Autodesk Fusion 360 part; units mm, degrees
sketch "base plate" plane through (0, 0, 0) normal (0, 0, 1) x (1, 0, 0)
  line L0 (-228.6, 228.6) -> (228.6, 228.6)
  line L1 (228.6, 228.6) -> (228.6, -228.6)
  line L2 (228.6, -228.6) -> (-228.6, -228.6)
  line L3 (-228.6, -228.6) -> (-228.6, 228.6)
  line L4 (-228.6, 228.6) -> (228.6, -228.6) construction
  line L5 (228.6, 228.6) -> (-228.6, -228.6) construction
  dimension "d1" = 457.2
  dimension "d2" = 457.2
extrude "Extrude1" add sketch "base plate" along normal blind 12.7 makes body 1
sketch "cylinder components" plane through (0, 0, 12.7) normal (0, 0, 1) x (-1, 0, 0)
  line L0 (228.6, 228.6) -> (-228.6, 228.6)
  line L1 (-228.6, 228.6) -> (-228.6, -228.6)
  line L2 (-228.6, -228.6) -> (228.6, -228.6)
  line L3 (228.6, -228.6) -> (228.6, 228.6)
  line L4 (25.4, -114.3) -> (-50.8, -114.3)
  line L5 (-50.8, -114.3) -> (-50.8, 76.2)
  line L6 (-50.8, 76.2) -> (25.4, 76.2)
  line L7 (25.4, 76.2) -> (25.4, -114.3)
  line L8 (-168.91, -76.2) -> (-226.06, -76.2)
  line L9 (-226.06, -76.2) -> (-226.06, -19.05)
  line L10 (-226.06, -19.05) -> (-168.91, -19.05)
  line L11 (-168.91, -19.05) -> (-168.91, -76.2)
  line L12 (0, -254) -> (0, 228.6) construction
  line L13 (25.4, 114.3) -> (-31.75, 114.3)
  line L14 (-31.75, 114.3) -> (-31.75, 171.45)
  line L15 (-31.75, 171.45) -> (25.4, 171.45)
  line L16 (25.4, 171.45) -> (25.4, 114.3)
  line L17 (-50.8, -64.605) -> (-168.91, -64.605)
  line L18 (-168.91, -64.605) -> (-168.91, -56.223)
  line L19 (-168.91, -56.223) -> (-50.8, -56.223)
  line L20 (-50.8, -56.223) -> (-50.8, -64.605)
  line L21 (226.06, -76.2) -> (168.91, -76.2)
  line L22 (168.91, -76.2) -> (168.91, -19.05)
  line L23 (168.91, -19.05) -> (226.06, -19.05)
  line L24 (226.06, -19.05) -> (226.06, -76.2)
  line L25 (25.4, -66.1774) -> (168.91, -66.1774)
  line L26 (168.91, -66.1774) -> (168.91, -57.7954)
  line L27 (168.91, -57.7954) -> (25.4, -57.7954)
  line L28 (25.4, -57.7954) -> (25.4, -66.1774)
  line L29 (9.064, 76.2) -> (-9.97, 76.2)
  line L30 (-9.97, 76.2) -> (-9.97, 114.3)
  line L31 (-9.97, 114.3) -> (9.064, 114.3)
  line L32 (9.064, 114.3) -> (9.064, 76.2)
  dimension "d5" = 76.2
  dimension "d6" = 190.5
  dimension "d9" = 57.15
  dimension "d10" = 57.15
  dimension "d13" = 2.54
  dimension "d14" = 247.65
  dimension "d22" = 57.15
  dimension "d23" = 57.15
  dimension "d24" = 38.1
  dimension "d25" = 57.15
  dimension "d26" = 196.85
  dimension "d29" = 8.382
  dimension "d30" = 118.11
  dimension "d31" = 57.15
  dimension "d32" = 57.15
  dimension "d33" = 247.65
  dimension "d34" = 2.54
  dimension "d35" = 8.382
extrude "Extrude3" add sketch "cylinder components" along normal blind 15.24 contours L4 L5 L6 L7 L20 L28 L29 bodies 1
sketch "clip retention" plane through (0, 0, 27.94) normal (0, 0, 1) x (-1, 0, 0)
  line L0 (25.4, -114.3) -> (25.4, 76.2)
  line L1 (25.4, 76.2) -> (-50.8, 76.2)
  line L2 (-50.8, 76.2) -> (-50.8, -114.3)
  line L3 (-50.8, -114.3) -> (25.4, -114.3)
  line L4 (25.4, -50.8) -> (12.7, -50.8)
  line L5 (12.7, -50.8) -> (-12.7, -76.2)
  line L6 (-12.7, -76.2) -> (-38.1, -50.8)
  line L7 (-38.1, -50.8) -> (-50.8, -50.8)
  line L8 (-50.8, -114.3) -> (25.4, -114.3)
  line L9 (25.4, -50.8) -> (25.4, -114.3)
  line L10 (19.05, -25.4) -> (-44.45, -25.4)
  line L11 (-44.45, -25.4) -> (-44.45, 25.4)
  line L12 (-44.45, 25.4) -> (19.05, 25.4)
  line L13 (19.05, 25.4) -> (19.05, -25.4)
  line L14 (-50.8, -50.8) -> (-50.8, -52.9164)
  line L15 (-50.8, -50.8) -> (-50.8, -114.3)
  point P0 (-12.7, -76.2)
  point P1 (-50.8, -114.3)
  point P2 (25.4, -114.3)
  dimension "d41" = 50.8
  dimension "d42" = 6.35
  dimension "d43" = 6.35
  dimension "d44" = 50.8
extrude "Extrude4" add sketch "cylinder components" along normal blind 6.35 contours L21 L22 L23 L24 L26 | L8 L9 L10 L11 L18 | L13 L14 L15 L16 L31 bodies 1
extrude "Extrude5" add sketch "cylinder components" along normal blind 8.382 contours L7 L22 L25 L26 L27 L28 | L5 L11 L17 L18 L19 L20 | L6 L13 L29 L30 L31 L32 bodies 1
extrude "Extrude6" add sketch "clip retention" along normal blind 15.24 contours L0 L2 L3 L4 L5 L6 L7 L8 L9 L14 L15 | L10 L11 L12 L13 bodies 1
sketch "clip hammer post cut out" plane through (0, 0, 43.18) normal (0, 0, 1) x (-1, 0, 0)
  line L0 (19.05, 25.4) -> (-44.45, 25.4)
  line L1 (-44.45, 25.4) -> (-44.45, -25.4)
  line L2 (-44.45, -25.4) -> (19.05, -25.4)
  line L3 (19.05, -25.4) -> (19.05, 25.4)
  line L4 (0, -12.7) -> (-25.4, -12.7)
  line L5 (-25.4, -12.7) -> (-25.4, 25.4)
  line L6 (-25.4, 25.4) -> (0, 25.4)
  line L7 (0, 25.4) -> (0, -12.7)
  line L8 (-7.2894, -38.3626) -> (-18.4141, -38.3626)
  line L9 (-18.4141, -38.3626) -> (-18.4141, -12.7)
  line L10 (-18.4141, -12.7) -> (-7.2894, -12.7)
  line L11 (-7.2894, -12.7) -> (-7.2894, -38.3626)
  dimension "d47" = 38.1
extrude "Extrude7" cut sketch "clip hammer post cut out" against normal blind 12.7 contours L0 L4 L5 L6 L7 L10 | L2 L8 L9 L11 | L2 L4 L9 L10 L11 bodies 1
sketch "clip hammer post" plane through (0, 0, 30.48) normal (0, 0, 1) x (-1, 0, 0)
  line L0 (-18.4141, -25.4) -> (-7.2894, -25.4)
  line L1 (-7.2894, -25.4) -> (-7.2894, -12.7)
  line L2 (-7.2894, -12.7) -> (0, -12.7)
  line L3 (0, -12.7) -> (0, 25.4)
  line L4 (0, 25.4) -> (-25.4, 25.4)
  line L5 (-25.4, 25.4) -> (-25.4, -12.7)
  line L6 (-25.4, -12.7) -> (-18.4141, -12.7)
  line L7 (-18.4141, -12.7) -> (-18.4141, -25.4)
  line L8 (-7.2894, -25.4) -> (-7.2894, -12.7)
  line L9 (0, -12.7) -> (0, 25.4)
  line L10 (-25.4, 25.4) -> (-25.4, -12.7)
  line L11 (-18.4141, -12.7) -> (-18.4141, -25.4)
  line L12 (-7.2894, -25.4) -> (-18.4141, -25.4)
  line L13 (0, 25.4) -> (-25.4, 25.4)
extrude "Extrude8" add sketch "clip hammer post" along normal blind 15.24 bodies 1
sketch "clip hammer" plane through (0, 0, 30.48) normal (0, 0, 1) x (1, 0, 0)
  line L0 (-5.08, 38.1) -> (30.8356, 38.1)
  line L1 (30.8356, 38.1) -> (12.8778, 65.9493)
  line L2 (12.8778, 65.9493) -> (-5.08, 38.1)
  dimension "d54" = 35.9156
extrude "Extrude9" add sketch "clip hammer" along normal blind 15.24 separate body makes body 2
sketch "Sketch7" plane through (0, 0, 27.94) normal (0, 0, 1) x (-1, 0, 0)
  line L0 (-50.8, -50.8) -> (-38.1, -50.8)
  line L1 (-38.1, -50.8) -> (-12.7, -76.2)
  line L2 (-12.7, -76.2) -> (12.7, -50.8)
  line L3 (12.7, -50.8) -> (25.4, -50.8)
  line L4 (25.4, -50.8) -> (25.4, 76.2)
  line L5 (25.4, 76.2) -> (-50.8, 76.2)
  line L6 (-50.8, 76.2) -> (-50.8, -50.8)
  line L7 (19.05, 25.4) -> (19.05, -25.4)
  line L8 (19.05, -25.4) -> (-44.45, -25.4)
  line L9 (-44.45, -25.4) -> (-44.45, 25.4)
  line L10 (-44.45, 25.4) -> (19.05, 25.4)
  line L11 (-6.5765, -38.1) -> (-18.4141, -38.1)
  line L12 (-18.4141, -38.1) -> (-18.4141, -25.4)
  line L13 (-18.4141, -25.4) -> (-6.5765, -25.4)
  line L14 (-6.5765, -25.4) -> (-6.5765, -38.1)
  line L15 (5.08, -38.1) -> (-30.8356, -38.1)
  point P0 (-18.4141, -25.4)
extrude "Extrude10" add sketch "Sketch7" along normal blind 15.24 contours L8 L11 L12 L13 L14 L15 bodies 1 2
Could you check a few things on this model? Use its own coordinates, in mm. A direction names the side the tool comes from. Coordinates: 2 decimals unless noted, no trailing zeros. Loops run counter-clockwise (first coordinate to the right, second up) from the corner with the lowest first, then second, coordinate; pieces in that order, holes last. Notation, with made-up numbers: (-6.5, 48.25) -> (16.5, 48.25) arc R20 ccw to (16.5, 61.25) -> close; hole circle Ø9 at (47, 26.25). An arc over 180 degrees is marked (long way). Answer in a Markdown table with one row per item.
(1) Imagine slicing it at C-C (y = -11). List the corners of the cut face in (x, z) for me.
Results found:
| item | result |
|---|---|
| outline | (-228.6, 0) -> (228.6, 0) -> (228.6, 12.7) -> (50.8, 12.7) -> (50.8, 27.94) -> (44.45, 27.94) -> (44.45, 43.18) -> (25.4, 43.18) -> (25.4, 45.72) -> (0, 45.72) -> (0, 43.18) -> (-19.05, 43.18) -> (-19.05, 27.94) -> (-25.4, 27.94) -> (-25.4, 12.7) -> (-228.6, 12.7) -> close |
(2) If I drill on probe 1 along X at (y, z) = (57, 15); probe 2 along Y at (x, z) = (30, 43); probe 3 along Y at (x, z) = (44, 43), over which ranges is the centre line in solid material (lowest first)?
Results found:
| item | result |
|---|---|
| probe 1 | x = -226.06 to -168.91, -25.4 to 226.06 |
| probe 2 | y = -25.4 to 25.4, 38.1 to 39.4, 58.9 to 114.3 |
| probe 3 | y = -25.4 to 25.4, 50.8 to 114.3 |
(3) Will these pins go through, and if not, where does the flat tip stop? pin 1 Ø2 at (y, z) = (21.5, 44.5) entering from +X; pin 2 Ø1.9 at (x, z) = (203.5, 17.5) entering from +Y; pin 3 Ø7 at (x, z) = (-16, 16.5) entering from +Y.
Results found:
| item | result |
|---|---|
| pin 1 | stops at x = 18.41 |
| pin 2 | stops at y = 76.2 |
| pin 3 | stops at y = 114.3 |
(4) Imagine slicing it at A-A (y = -88.5). List the corners of the cut face in (x, z) for me, plus the area to 3 significant figures.
Results found:
| item | result |
|---|---|
| outline | (-228.6, 0) -> (228.6, 0) -> (228.6, 12.7) -> (9.97, 12.7) -> (9.97, 21.08) -> (-9.06, 21.08) -> (-9.06, 12.7) -> (-228.6, 12.7) -> close |
| area | 5,970 mm^2 |
(5) For faces 4 (the face through (12, 114.3, 28)), 5 (the face through (44.45, 0, 35)), 6 (the face through (4.025, 52.22, 37.993)), which set-ups out of +Z, -Z, +X, -X, +Y, -Y let a thin tool reach every point of the face, with its end or its side?
Results found:
| item | result |
|---|---|
| face 4 | +Z, +X, -X, +Y |
| face 5 | +Z, +X, -Y |
| face 6 | +Z |
(6) Imagine slicing it at D-D (y = 179.5). List the corners of the cut face in (x, z) for me.
Results found:
| item | result |
|---|---|
| outline | (-228.6, 0) -> (228.6, 0) -> (228.6, 12.7) -> (-228.6, 12.7) -> close |
(7) Imagine slicing it at B-B (x = -46). List the corners of the cut face in (y, z) for me, plus the area to 3 significant figures.
Results found:
| item | result |
|---|---|
| outline | (-228.6, 0) -> (228.6, 0) -> (228.6, 12.7) -> (66.18, 12.7) -> (66.18, 21.08) -> (57.8, 21.08) -> (57.8, 12.7) -> (-228.6, 12.7) -> close |
| area | 5,880 mm^2 |
(8) Thinking about a two-plate mould opening in Y: for faces 1 (the face through (-25.4, 39, 24)), 2 (the face through (13, -25.4, 37)), 3 (the face through (25.2, 63.7, 35.5)), which applies, released by +Y, released by -Y, zero draft, split by the parting line, or undercut?
Results found:
| item | result |
|---|---|
| face 1 | zero draft |
| face 2 | released by -Y |
| face 3 | undercut |
